Work out the finished part from the listing and answer in its coordinate system (mm). Round coordinates to 2 decimals unless told otherwise and drop trailing zeros. Order: outer loops, then holes, each group sorted by start corner. A loop starts at its lowest first (then second) coordinate and runs counter-clockwise, first axis right, second up.
Autodesk Inventor part; units mm, degrees
ref_plane "YZ Plane" through (0, 0, 0) normal (1, 0, 0) x (0, 1, 0)
ref_plane "XZ Plane" through (0, 0, 0) normal (0, 1, 0) x (-1, 0, 0)
ref_plane "XY Plane" through (0, 0, 0) normal (0, 0, 1) x (1, 0, 0)
sketch "スケッチ1" plane through (0, 0, 0) normal (0, 1, 0) x (-1, 0, 0)
  line L0 (-20, 20) -> (20, 20)
  line L1 (20, 20) -> (20, -20)
  line L2 (20, -20) -> (-20, -20)
  line L3 (-20, -20) -> (-20, 20)
  point P0 (0, 0)
  dimension "d0" = 40
  dimension "d2" = 40
  dimension "d3" = 20
  dimension "d4" = 20
extrude "押し出し1" add sketch "スケッチ1" along normal blind 2
sketch "スケッチ2" plane through (0, 2, 0) normal (0, 1, 0) x (1, 0, 0)
  line L0 (-20, -20) -> (20, -20)
  line L1 (20, -20) -> (20, 20)
  line L2 (20, 20) -> (-20, 20)
  line L3 (-20, 20) -> (-20, -20)
  circle A0 centre (-15, -15) radius 3
  circle A1 centre (-5, -15) radius 3
  circle A2 centre (5, -15) radius 3
  circle A3 centre (15, -15) radius 3
  circle A4 centre (-15, -5) radius 3
  circle A5 centre (-15, 5) radius 3
  circle A6 centre (-15, 15) radius 3
  circle A7 centre (-5, -5) radius 3
  circle A8 centre (-5, 5) radius 3
  circle A9 centre (-5, 15) radius 3
  circle A10 centre (5, -5) radius 3
  circle A11 centre (15, -5) radius 3
  circle A12 centre (15, 5) radius 3
  circle A13 centre (5, 5) radius 3
  circle A14 centre (5, 15) radius 3
  circle A15 centre (15, 15) radius 3
  point P0 (0, 0)
  dimension "d7" = 6
  dimension "d9" = 10
  dimension "d10" = 10
  dimension "d11" = 10
  dimension "d12" = 5
  dimension "d13" = 5
  dimension "d14" = 5
  dimension "d15" = 5
  dimension "d16" = 5
  dimension "d17" = 10
  dimension "d18" = 10
  dimension "d19" = 10
  dimension "d20" = 5
  dimension "d21" = 5
  dimension "d22" = 5
  dimension "d23" = 10
  dimension "d24" = 10
  dimension "d25" = 10
  dimension "d26" = 10
  dimension "d27" = 10
  dimension "d28" = 10
  dimension "d29" = 10
  dimension "d30" = 10
  dimension "d31" = 10
  dimension "d32" = 10
  dimension "d33" = 10
  dimension "d34" = 10
  dimension "d35" = 10
  dimension "d36" = 10
  dimension "d37" = 10
  dimension "d38" = 10
  dimension "d39" = 10
  dimension "d40" = 10
extrude "押し出し2" add sketch "スケッチ2" along normal blind 0.5
properties part number "fai6_sikiita"
Item 1: Find the intervals of material crossed by line 1 along Z through (x, y) = (15, 2.15); line 2 along Z through (x, y) = (-12.5, 2.3), in increasing order.
Item 2: For a pull along Z with two mould halves and no side action, classify faces 1 (the face through (0, 2.5, 0)), 2 (the face through (5, 2, 5)) as released by +Z, released by -Z, zero draft, split by the parting line, or undercut.
Item 3: Given pin 1 (3 mm diameter, centred on x = -5.5, z = 14.5, fed in from +Y), flat-ended and moving along its own axis, determine where the tip first touches the part or whether it passes through.
Item 4: Find section B-B (x = -5). Write down the section's boundary in (y, z), plus the area to 3 significant figures.
Item 5: Find section A-A (z = 15). Write down the section's boundary in (x, y).
Model answer:
1. line 1: z = -20 to -18, -12 to -8, -2 to 2, 8 to 12, 18 to 20
1. line 2: z = -20 to -16.66, -13.34 to -6.66, -3.34 to 3.34, 6.66 to 13.34, 16.66 to 20
2. face 1: zero draft
2. face 2: undercut
3. pin 1: stops at y = 2
4. outline: (0, -20) - (2.5, -20) - (2.5, -18) - (2, -18) - (2, -12) - (2.5, -12) - (2.5, -8) - (2, -8) - (2, -2) - (2.5, -2) - (2.5, 2) - (2, 2) - (2, 8) - (2.5, 8) - (2.5, 12) - (2, 12) - (2, 18) - (2.5, 18) - (2.5, 20) - (0, 20) - close
4. area: 88.0 mm2
5. outline: (-20, 0) - (20, 0) - (20, 2.5) - (18, 2.5) - (18, 2) - (12, 2) - (12, 2.5) - (8, 2.5) - (8, 2) - (2, 2) - (2, 2.5) - (-2, 2.5) - (-2, 2) - (-8, 2) - (-8, 2.5) - (-12, 2.5) - (-12, 2) - (-18, 2) - (-18, 2.5) - (-20, 2.5) - close
